Source: three-view drawing plus pictorial views. Frame: mm from the lowest corner of the part. A direction names the side the tool comes from. Coordinates: 2 decimals unless noted, no trailing zeros. Write each loop counter-clockwise with the first axis right and the second up, starting at its lowest first coordinate (ties: lowest second). Pieces come first, ordered by that corner, then holes. Notation, with made-up numbers: M 68,-1 L 78,-1 A28 ccw 78,21 Z; hole C 89.25,-5 d8. An arc over 180 degrees is marked long. Use CSV: the item, a comma, the result in double quotes.
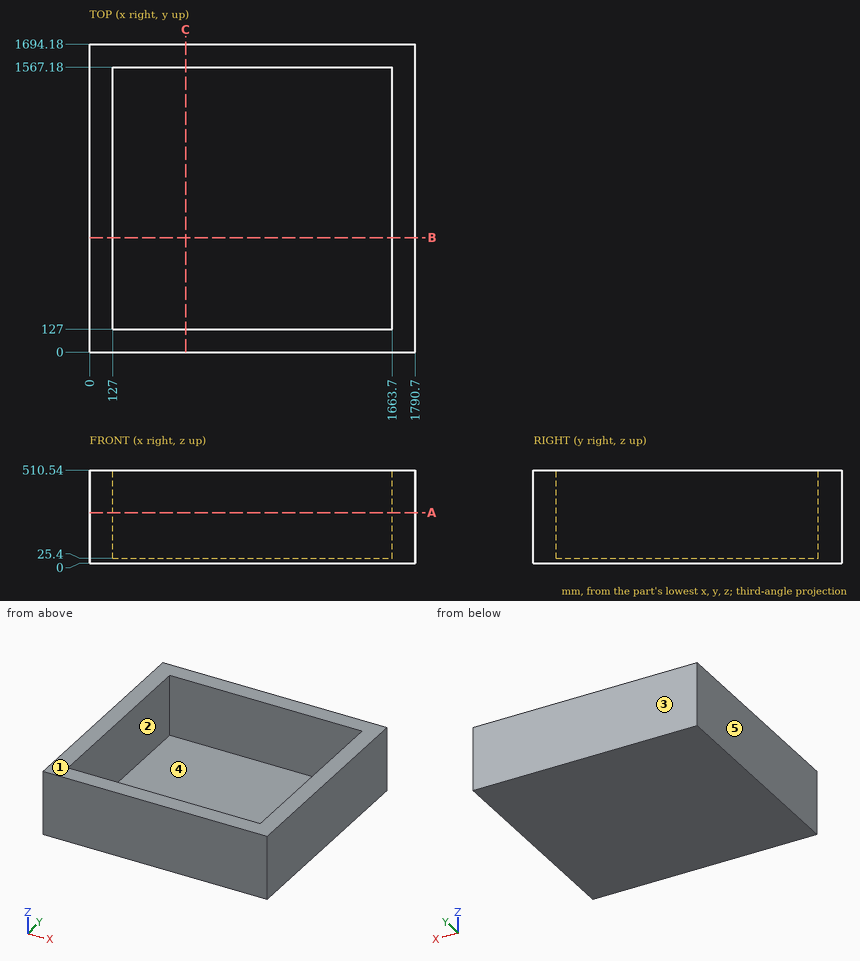
1. Access query for the marked faces 1 and 2. Directions: +Z, -Z, +X, -X, +Y, -Y. A direction counts if a zero-diameter tool reaches every point of the face in a straight line with its end or side. Return the directions, or none.
Resolved:
face 1,"+Z, +X, -X, +Y, -Y"
face 2,"+Z"
2. Section C-C (x = 528.5). Return loops of the section in (y, z).
Resolved:
outline,"M 0,0 L 1694.18,0 L 1694.18,510.54 L 1567.18,510.54 L 1567.18,25.4 L 127,25.4 L 127,510.54 L 0,510.54 Z"
3. Section B-B (y = 630.5). Return loops of the section in (x, z).
Resolved:
outline,"M 0,0 L 1790.7,0 L 1790.7,510.54 L 1663.7,510.54 L 1663.7,25.4 L 127,25.4 L 127,510.54 L 0,510.54 Z"
4. Material intervals for line 1 (X direction, y = 1319.5, z = 38.5); line 2 (Y direction, x = 1511, z = 449); line 3 (Z direction, x = 1263.5, y = 342), sorted ascending. Write a range as [from, to].
Resolved:
line 1,"x = [0, 127], [1663.7, 1790.7]"
line 2,"y = [0, 127], [1567.18, 1694.18]"
line 3,"z = [0, 25.4]"
5. Section A-A (z = 277.5). Return loops of the section in (x, y), then the cut area to 3 significant figures.
Resolved:
outline,"M 0,0 L 1790.7,0 L 1790.7,1694.18 L 0,1694.18 Z; hole M 127,127 L 1663.7,127 L 1663.7,1567.18 L 127,1567.18 Z"
area,"821,000 mm^2"
6. Mould query, pull axis Y, two halves, no side actions, for the marked faces 3, 4 and 5. Classes: pulls with the +Y half, pulls with the -Y half, needs draft (parallel to the pull), parting line crosses it, or undercut.
Resolved:
face 3,"pulls with the +Y half"
face 4,"undercut"
face 5,"needs draft"
